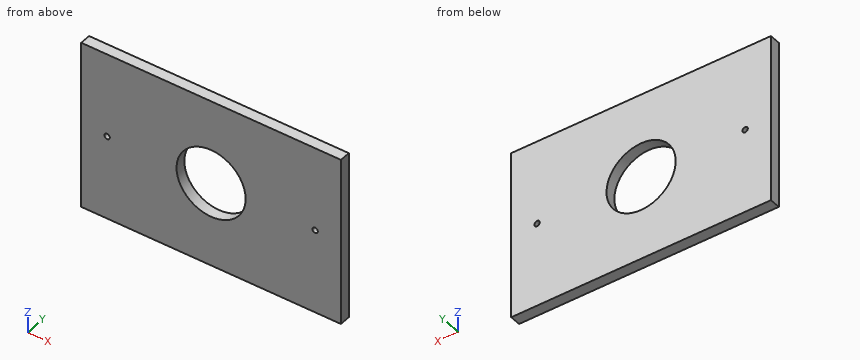
```python
from build123d import *

# Parameters (mm, degrees)
SKETCH1_W           = 152.7
SKETCH1_H           = 100
BOSS_EXTRUDE1_DEPTH = 6.35
SKETCH2_R           = 20.32
CUT_EXTRUDE1_DEPTH  = 10
SKETCH3_R           = 1.5875
CUT_EXTRUDE2_DEPTH  = 10


with BuildPart() as part:
    # Sketch1 → Boss-Extrude1 (new body)
    with BuildSketch(Plane(origin=(0, 0, 0), x_dir=(1, 0, 0), z_dir=(0, 1, 0))):
        with Locations((76.35, 50)):
            Rectangle(SKETCH1_W, SKETCH1_H)
    extrude(amount=BOSS_EXTRUDE1_DEPTH)

    # Sketch2 → Cut-Extrude1 (cut)
    with BuildSketch(Plane(origin=(0, 6.35, 0), x_dir=(1, 0, 0), z_dir=(0, 1, 0))):
        with Locations(Location((76.35, 50, 0), (0, 0, 270))):
            Circle(SKETCH2_R)
    extrude(amount=-CUT_EXTRUDE1_DEPTH, mode=Mode.SUBTRACT)

    # Sketch3 → Cut-Extrude2 (cut)
    with BuildSketch(Plane(origin=(0, 6.35, 0), x_dir=(1, 0, 0), z_dir=(0, 1, 0))):
        with Locations(Location((15.2, 50, 0), (0, 0, 270))):
            Circle(SKETCH3_R)
        with Locations(Location((137.5, 50, 0), (0, 0, 270))):
            Circle(SKETCH3_R)
    extrude(amount=-CUT_EXTRUDE2_DEPTH, mode=Mode.SUBTRACT)


solid = part.part
```
CAD build for the part. Positions are in the model's coordinates, mm. Give positions to 0.01 mm unless a question says otherwise; leave off trailing zeros. Write each loop counter-clockwise with the first axis right and the second up, starting at its lowest first coordinate (ties: lowest second). Pieces come first, ordered by that corner, then holes. Notation, with made-up numbers: (77, -28) -> (129, -28) arc R18 cw to (129, 1) -> close; hole circle Ø11 at (62, 80.5). An arc over 180 degrees is marked (long way). Write each question's results on one line, items separated by ' | '.
1. Cut at C-C, the plane y = 3.75. Give the number of separate pieces and of enclosed holes in the cut face, then the cut area to 3 significant figures.
Geometry check:
separate pieces: 1 | enclosed holes: 3 | area: 14,000 mm²
2. Cut at B-B, the plane z = -50. Write the cut outline in (x, y), then the cut area to 3 significant figures.
Geometry check:
outline: (0, 0) -> (13.61, 0) -> (13.61, 6.35) -> (0, 6.35) -> close; (16.79, 0) -> (56.03, 0) -> (56.03, 6.35) -> (16.79, 6.35) -> close; (96.67, 0) -> (135.91, 0) -> (135.91, 6.35) -> (96.67, 6.35) -> close; (139.09, 0) -> (152.7, 0) -> (152.7, 6.35) -> (139.09, 6.35) -> close | area: 671 mm²
3. Wall check: probe 1 along X at (y, z) = (2.75, -50); probe 2 along Z at (x, y) = (137.5, 2.75); probe 3 along Z at (x, y) = (77.5, 4.25). Give the ranges that are in metal, low to high. Write a range as [from, to].
Geometry check:
probe 1: [0, 13.61], [16.79, 56.03], [96.67, 135.91], [139.09, 152.7] | probe 2: [-100, -51.59], [-48.41, 0] | probe 3: [-100, -70.29], [-29.71, 0]
4. Cut at D-D, the plane z = -61. Write the cut outline in (x, y), then the cut area to 3 significant figures.
Geometry check:
outline: (0, 0) -> (59.26, 0) -> (59.26, 6.35) -> (0, 6.35) -> close; (93.44, 0) -> (152.7, 0) -> (152.7, 6.35) -> (93.44, 6.35) -> close | area: 753 mm²
5. Cut at A-A, the plane x = 137.5. Write the cut outline in (y, z).
Geometry check:
outline: (0, -100) -> (6.35, -100) -> (6.35, -51.59) -> (0, -51.59) -> close; (0, -48.41) -> (6.35, -48.41) -> (6.35, 0) -> (0, 0) -> close
